Build history of the part. All positions in model axes, mm. Face numbers are marked on the shaded views. A direction names the side the tool comes from. Coordinates: 2 decimals unless noted, no trailing zeros. Order: outer loops, then holes, each group sorted by start corner. A loop starts at its lowest first (then second) coordinate and runs counter-clockwise, first axis right, second up. Notation, with made-up numbers: M 16,-15.75 L 64,-15.75 A28 cw 64,14.25 Z; hole C -32.5,19 d8. An arc over 180 degrees is marked long. Use a Markdown table: item, result. Add a question column.
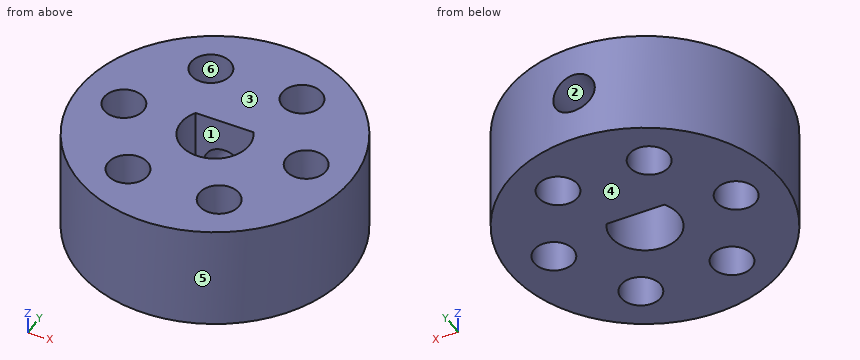
Autodesk Inventor part; units mm, degrees
ref_plane "YZ Plane" through (0, 0, 0) normal (1, 0, 0) x (0, 1, 0)
ref_plane "XZ Plane" through (0, 0, 0) normal (0, 1, 0) x (-1, 0, 0)
ref_plane "XY Plane" through (0, 0, 0) normal (0, 0, 1) x (1, 0, 0)
sketch "Sketch9" plane through (0, 0, 0) normal (0, 0, 1) x (1, 0, 0)
  circle A0 centre (0, 0) radius 4.125 construction
  circle A1 centre (0, 0) radius 16.5
  circle A2 centre (11, 0) radius 2.4
  circle A3 centre (5.5, 9.5263) radius 2.4
  circle A4 centre (-5.5, 9.5263) radius 2.4
  line L0 (-3.4894, 2.2) -> (3.4894, 2.2)
  arc A5 (-3.4894, 2.2) -> (3.4894, 2.2) centre (0, 0) ccw
  circle A6 centre (-11, 0) radius 2.4
  circle A7 centre (-5.5, -9.5263) radius 2.4
  circle A8 centre (5.5, -9.5263) radius 2.4
  dimension "d25" = 8.25
  dimension "d26" = 33
  dimension "d27" = 4.8
  dimension "d31" = 360
  dimension "d33" = 2.2
  dimension "d36" = 11
extrude "Extrusion8" add sketch "Sketch9" along normal blind 12.7
sketch "Sketch10" plane through (-3.4894, 2.2, 0) normal (0, -1, 0) x (1, 0, 0)
  line L0 (6.9787, 0) -> (0, 0)
  line L1 (6.9787, 0) -> (6.9787, 12.7)
  line L2 (0, 12.7) -> (6.9787, 12.7)
  line L3 (0, 0) -> (0, 12.7)
  circle A0 centre (3.4894, 6.35) radius 2.5
  point P0 (3.4894, 0)
  point P1 (3.4894, 12.7)
  point P2 (0, 6.35)
  dimension "d37" = 5
extrude "Extrusion9" cut sketch "Sketch10" against normal through all contours A0
properties part number "AA055" material "Aluminum 6061"
(1) Mould opens along X. For the marked faces 4, 5 and 6 say: released by +X, released by -X, zero draft, split by the parting line, or undercut.
(2) Slice it at D-D on y = 0. Give the cut face in (x, z).
(3) Slice it at B-B on y = 9. Give the cut face in (x, z), and give its area (3 significant figures).
(4) Drop flat-ended pins along their axis: P1, Ø2, axis at y = -2.5, z = 8.5, coming from the +X side; P2, Ø1, axis at x = -6, z = 9.5, coming from the +Y side; P3, Ø2, axis at y = 7.5, z = 7.5, coming from the +X side. Give the stop position or say it passes through.
(5) Slice it at C-C on z = 5.5. Give the cut face in (x, y).
(6) Which spindle directions (+Z, -Z, +X, -X, +Y, -Y) get a long thin tool onto all of the face, cutting with end or side? Do the marked faces 1, 2 and 3. Say none if no direction does.
(7) Slice it at A-A on x = 0. Give the cut face in (y, z).
(8) Drill centre lines: line 1 along Z through (x, y) = (0, 12.5); line 2 along Y through (x, z) = (-5.5, 4); line 3 along X through (y, z) = (-9.5, 12). Where is each one in solid material? Low to high. Write a range as from..to.
Solutions:
| question | item | result |
|---|---|---|
| 1 | face 4 | zero draft |
| 1 | face 5 | split by the parting line |
| 1 | face 6 | undercut |
| 2 | outline | M -16.5,0 L -13.4,0 L -13.4,12.7 L -16.5,12.7 Z; M -8.6,0 L -4.13,0 L -4.13,12.7 L -8.6,12.7 Z; M 4.13,0 L 8.6,0 L 8.6,12.7 L 4.13,12.7 Z; M 13.4,0 L 16.5,0 L 16.5,12.7 L 13.4,12.7 Z |
| 3 | outline | M -13.83,0 L -7.84,0 L -7.84,12.7 L -13.83,12.7 Z; M -3.16,0 L 3.16,0 L 3.16,12.7 L -3.16,12.7 Z; M 7.84,0 L 13.83,0 L 13.83,12.7 L 7.84,12.7 Z; hole C 0,6.35 d5 |
| 3 | area | 213 mm² |
| 4 | P1 | x = 16.43 |
| 4 | P2 | y = 15.56 |
| 4 | P3 | x = 15.17 |
| 5 | outline | M -3.49,2.2 L -2.35,2.2 L -2.35,16.33 A16.5 ccw long 2.35,16.33 L 2.35,2.2 L 3.49,2.2 A4.13 cw long Z; hole C -11,0 d4.8; hole C -5.5,-9.53 d4.8; hole C -5.5,9.53 d4.8; hole C 5.5,-9.53 d4.8; hole C 5.5,9.53 d4.8; hole C 11,0 d4.8 |
| 6 | face 1 | +Z, -Z |
| 6 | face 2 | +Y |
| 6 | face 3 | +Z, +X, -X, +Y, -Y |
| 7 | outline | M -16.5,0 L -4.13,0 L -4.13,12.7 L -16.5,12.7 Z; M 2.2,0 L 16.5,0 L 16.5,3.85 L 2.2,3.85 Z; M 2.2,8.85 L 16.5,8.85 L 16.5,12.7 L 2.2,12.7 Z |
| 8 | line 1 | 0..3.85, 8.85..12.7 |
| 8 | line 2 | -15.56..-11.93, -7.13..7.13, 11.93..15.56 |
| 8 | line 3 | -13.49..-7.9, -3.1..3.1, 7.9..13.49 |
